Verification items for the finished model (mm, model axes). A direction names the side the tool comes from. Round coordinates to 2 decimals unless told otherwise and drop trailing zeros. Write each loop counter-clockwise with the first axis right and the second up, starting at its lowest first coordinate (ties: lowest second). Pieces come first, ordered by that corner, then holes. Notation, with made-up numbers: (-22.5, 84) - (8.5, 84) arc R25 ccw to (8.5, 101) - close; hole circle Ø9 at (27, 1). An arc over 180 degrees is marked (long way). Answer as a JSON object with one key per item and string values. Group by question number.
1) Set-up check for faces 4 (the flat face through (0, -3, -6)), 5 (the flat face through (12.862, 3, -6)), 6 (the flat face through (12.862, 3, 6)), 7 (the flat face through (0, 3, 6)): record each of +Z, -Z, +X, -X, +Y, -Y from which the full face is reachable in a straight line by a thin tool's end or side.
2) Go/stop test with flat-tipped pins: pin 1 Ø6 at (x, z) = (110.5, -2.5) entering from +Y; pin 2 Ø3 at (x, y) = (103, -5) entering from -Z; pin 3 Ø0.5 at (y, z) = (-7, 0) entering from -X; pin 4 Ø4 at (x, z) = (9, -3.5) entering from +Y. Record where each tip stops, or that it passes through.
3) Thickness scan on line 1 (Y direction, x = 55.5, z = 3); line 2 (Z direction, x = 26, y = -5.25); line 3 (Y direction, x = 30, z = 1.75). Record the ranges inside material, lowest first.
4) Section check A-A (x = 97). Enter the section's corners in (y, z).
5) Section check B-B (z = -1.5). Enter the section's corners in (x, y), then the cut area to 3 significant figures.
6) Mould release check, pull along X, two halves, no side actions. Record for faces 1 (the flat face through (6.341, 5.474, 3.219)), 2 (the cylindrical face through (13.25, 1.38, -6.2)), 3 (the flat face through (-7.925, 0, 0)): +X half, -X half, draft (parallel to the pull), parting line (faces both ways), or undercut.
Autodesk Inventor part; units mm, degrees
ref_plane "YZ Plane" through (0, 0, 0) normal (1, 0, 0) x (0, 1, 0)
ref_plane "XZ Plane" through (0, 0, 0) normal (0, 1, 0) x (-1, 0, 0)
ref_plane "XY Plane" through (0, 0, 0) normal (0, 0, 1) x (1, 0, 0)
sketch "Sketch1" plane through (0, 0, 0) normal (1, 0, 0) x (0, 1, 0)
  line L0 (7.3323, 0) -> (3.6662, -6.35)
  line L1 (3.6662, -6.35) -> (-3.6662, -6.35)
  line L2 (-3.6662, -6.35) -> (-7.3323, 0)
  line L3 (-7.3323, 0) -> (-3.6662, 6.35)
  line L4 (-3.6662, 6.35) -> (3.6662, 6.35)
  line L5 (3.6662, 6.35) -> (7.3323, 0)
  circle A0 centre (0, 0) radius 6.35
  dimension "d0" = 12.7
extrude "Extrusion1" add sketch "Sketch1" along normal blind 26.2984
extrude "Extrusion2" add sketch "Sketch1" against normal blind 7.9248 contours A0
ref_plane "Work Plane1" through (0, 7.3323, 0) normal (0, 0, -1) x (1, 0, 0)
sketch "Sketch2" plane through (0, 7.3323, 0) normal (0, 0, -1) x (1, 0, 0)
  line L0 (0, 13.6823) -> (-7.9248, 13.6823)
  line L1 (0, 10.9985) -> (0, 14.6647)
  line L2 (0, 14.6647) -> (26.2984, 14.6647)
  line L3 (12.8618, 14.6647) -> (13.6492, 14.6647)
  line L4 (13.6492, 14.6647) -> (13.6492, 13.6823)
  line L5 (13.6492, 13.6823) -> (12.8618, 13.6823)
  line L6 (12.8618, 13.6823) -> (12.8618, 14.6647)
  line L7 (0, 7.3323) -> (26.2984, 7.3323)
  line L8 (26.2984, 3.6662) -> (26.2984, 10.9985)
  line L9 (26.2984, 14.6647) -> (26.2984, 10.9985)
  dimension "d7" = 0.7874
  dimension "d9" = 12.6492
revolve "Revolution1" cut sketch "Sketch2" angle 360 about axis through (0, 0, 0) along (1, 0, 0)
sketch "Sketch3" plane through (26.2984, 0, 0) normal (1, 0, 0) x (0, 0, -1)
  line L0 (6.35, 3.6662) -> (0, 7.3323)
  line L1 (0, 7.3323) -> (-6.35, 3.6662)
  line L2 (-6.35, 3.6662) -> (-6.35, -3.6662)
  line L3 (-6.35, -3.6662) -> (0, -7.3323)
  line L4 (0, -7.3323) -> (6.35, -3.6662)
  line L5 (6.35, -3.6662) -> (6.35, 3.6662)
  point P0 (0, 0)
extrude "Extrusion3" add sketch "Sketch3" along normal blind 100
properties part number "LongShaft"
Returned:
{
 "1": {"face 4": "-Z, -X, -Y", "face 5": "-Z, +Y", "face 6": "+Z, +Y", "face 7": "+Z, -X, +Y"},
 "2": {"pin 1": "y = 7.33", "pin 2": "z = -6.35", "pin 3": "x = 0", "pin 4": "y = 6.47"},
 "3": {"line 1": "-5.6 to 5.6", "line 2": "-3.61 to 3.61", "line 3": "-6.32 to 6.32"},
 "4": {"outline": "(-7.33, 0) - (-3.67, -6.35) - (3.67, -6.35) - (7.33, 0) - (3.67, 6.35) - (-3.67, 6.35) - close"},
 "5": {"outline": "(-7.92, -6.17) - (0, -6.17) - (0, -6.47) - (12.86, -6.47) - (12.86, -6.17) - (13.65, -6.17) - (13.65, -6.47) - (126.3, -6.47) - (126.3, 6.47) - (13.65, 6.47) - (13.65, 6.17) - (12.86, 6.17) - (12.86, 6.47) - (0, 6.47) - (0, 6.17) - (-7.92, 6.17) - close", "area": "1,730 mm2"},
 "6": {"face 1": "draft", "face 2": "undercut", "face 3": "-X half"}
}
